Work out the finished part from the listing and answer in its coordinate system (mm). Face numbers are marked on the shaded views. A direction names the side the tool comes from. Coordinates: 2 decimals unless noted, no trailing zeros. Loops run counter-clockwise (first coordinate to the right, second up) from the corner with the lowest first, then second, coordinate; pieces in that order, holes last. Notation, with made-up numbers: (-7, 24.5) - (0, 24.5) arc R26 cw to (0, 55.5) - close; hole circle Ø2 at (81.5, -25.75). An arc over 180 degrees is marked (long way). Write each question's results on one line, items separated by ' | '. Start each with the question number.
1. Which of the six approach directions +Z, -Z, +X, -X, +Y, -Y give full straight-line access (tool end or side, diameter ignored) to the marked faces 1 and 2?
2. A cutting plane is placed at C-C on x = 38. Determine the outline of the cut face in (y, z) (3 decimals), then the cut area to 3 significant figures.
3. A cutting plane is placed at B-B on z = -4.5. Determine the outline of the cut face in (x, y) (3 decimals), then the cut area to 3 significant figures.
4. Find the intervals of material crossed by line 1 along X through (y, z) = (10.25, -55); line 2 along X through (y, z) = (7, -43.5); line 3 along Z through (x, y) = (46.5, 1.5), in increasing order. Write a range as [from, to].
5. A cutting plane is placed at A-A on y = 15.75. Determine the outline of the cut face in (x, z) (3 decimals).
6. Each of these flat-tipped pins is pushed along its axis until it touches: P1, Ø1.5, axis at x = 21.5, z = -56, coming from the -Y side; P2, Ø1.5, axis at x = 6.5, y = 17.5, coming from the -Z side; P3, Ø3, axis at y = 11, z = -6, coming from the -X side; P4, Ø2, axis at x = 40.5, y = 4.5, coming from the -Z side. Where does it stop, or does it pass through?
from build123d import *

# Parameters (mm, degrees)
BOSS_EXTRUDE1_DEPTH = 22.225


with BuildPart() as part:
    # Sketch1 → Boss-Extrude1 (new body)
    with BuildSketch(Plane(origin=(0, 0, 0), x_dir=(1, 0, 0), z_dir=(0, 1, 0))):
        with BuildLine():
            Line((0, 63.5), (0, 9.525))
            Line((0, 9.525), (31.75, 9.525))
            Line((31.75, 9.525), (31.75, 0))
            Line((31.75, 0), (63.5, 0))
            ThreePointArc((63.5, 0), (44.901280605, 44.901280605), (0, 63.5))
        make_face()
    extrude(amount=BOSS_EXTRUDE1_DEPTH)


solid = part.part
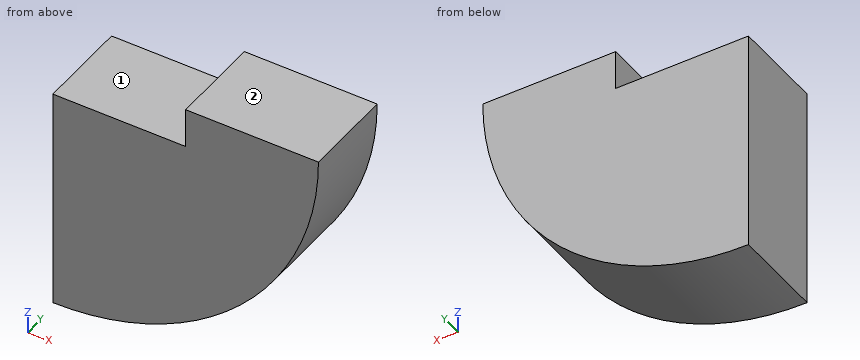
Values:
1) face 1: +Z, -X, +Y, -Y | face 2: +Z, +X, -X, +Y, -Y
2) outline: (0, -50.875) - (22.225, -50.875) - (22.225, 0) - (0, 0) - close | area: 1,130 mm^2
3) outline: (31.75, 0) - (63.34, 0) - (63.34, 22.225) - (31.75, 22.225) - close | area: 702 mm^2
4) line 1: [0, 31.74] | line 2: [0, 46.26] | line 3: [-43.24, 0]
5) outline: (0, -63.5) arc R63.5 ccw to (63.5, 0) - (31.75, 0) - (31.75, -9.525) - (0, -9.525) - close
6) P1: y = 0 | P2: z = -63.24 | P3: x = 31.75 | P4: z = -49.72
